```python
from build123d import *

# Parameters (mm, degrees)
PAD_DEPTH            = 42.5
SKETCH001_R          = 3.1
POCKET_DEPTH         = 27.001
POCKET_DEPTH_BACK    = -5.001
SKETCH002_R          = 2.6
SKETCH002_R_2        = 3.1
POCKET001_DEPTH      = 7.001
FILLET_R             = 2
SKETCH005_R          = 0.5
POCKET002_DEPTH      = 7.001
POCKET002_DEPTH_BACK = -27.001
SKETCH006_R          = 6
POCKET003_DEPTH      = 2


with BuildPart() as part:
    # Sketch → Pad (new body, symmetric)
    with BuildSketch(Plane.XZ):
        Polygon((-7, 5), (27, 5), (27, 0), (0, 0), (0, -27), (-7, -27), align=None)
    extrude(amount=PAD_DEPTH, both=True)

    # Sketch001 → Pocket (cut, two sides)
    with BuildSketch(Plane.XY) as pocket_sk:
        with Locations((15, -21)):
            Circle(SKETCH001_R)
        with Locations((15, 21)):
            Circle(SKETCH001_R)
    extrude(amount=-POCKET_DEPTH, mode=Mode.SUBTRACT)
    extrude(pocket_sk.sketch, amount=-POCKET_DEPTH_BACK, mode=Mode.SUBTRACT)

    # Sketch002 → Pocket001 (cut, through all)
    with BuildSketch(Plane.YZ):
        with Locations((-21, -15)):
            Circle(SKETCH002_R)
        with Locations((21, -15)):
            Circle(SKETCH002_R)
        with Locations((-35, -15)):
            Circle(SKETCH002_R_2)
        with Locations((35, -15)):
            Circle(SKETCH002_R_2)
    extrude(amount=-POCKET001_DEPTH, mode=Mode.SUBTRACT)

    # Sketch003 (on DatumPlane) → Groove (revolve, cut)
    with BuildSketch(Plane.XY.offset(-15)):
        Polygon((0, 21), (-5, 21), (0, 16), align=None)
    revolve(axis=Axis((0, 21, -15), (1, 0, 0)), mode=Mode.SUBTRACT)

    # Sketch004 (on DatumPlane) → Groove001 (revolve, cut)
    with BuildSketch(Plane.XY.offset(-15)):
        Polygon((-5, -21), (0, -21), (0, -16), align=None)
    revolve(axis=Axis((0, -21, -15), (1, 0, 0)), mode=Mode.SUBTRACT)

    # Fillet
    fillet_edges = [part.edges().sort_by_distance(p)[0] for p in [
        (-3.5, -42.5, -27),
        (-3.5, 42.5, -27),
        (10, -42.5, 5),
        (10, 42.5, 5),
    ]]
    fillet(fillet_edges, radius=FILLET_R)

    # Sketch005 → Pocket002 (cut, two sides)
    with BuildSketch(Plane.YZ) as pocket002_sk:
        with Locations((0, -27)):
            Circle(SKETCH005_R)
    extrude(amount=-POCKET002_DEPTH, mode=Mode.SUBTRACT)
    extrude(pocket002_sk.sketch, amount=-POCKET002_DEPTH_BACK, mode=Mode.SUBTRACT)

    # Sketch006 (on Face2 of Pocket002) → Pocket003 (cut)
    with BuildSketch(Plane(origin=(-7, 0, 0), x_dir=(0, 0, -1), z_dir=(-1, 0, 0))):
        with Locations((15, 35)):
            Circle(SKETCH006_R)
        with Locations((15, -35)):
            Circle(SKETCH006_R)
    extrude(amount=-POCKET003_DEPTH, mode=Mode.SUBTRACT)


solid = part.part
```
Check sheet for the modelled part. Datum: model origin and axes. Units: mm. A direction names the side the tool comes from. Round coordinates to 2 decimals unless told otherwise and drop trailing zeros. Write each loop counter-clockwise with the first axis right and the second up, starting at its lowest first coordinate (ties: lowest second). Pieces come first, ordered by that corner, then holes. Notation, with made-up numbers: (80.25, -9) -> (104.25, -9) arc R15 cw to (104.25, 9) -> close; hole circle Ø6 at (41.25, 33.25). An arc over 180 degrees is marked (long way). Put each result on its own line as item: value.
(1) Sectioned sample at C-C (y = -35). Enter the section's corners in (x, z).
Values found:
outline: (-7, -27) -> (0, -27) -> (0, -18.1) -> (-5, -18.1) -> (-5, -21) -> (-7, -21) -> close; (-7, -9) -> (-5, -9) -> (-5, -11.9) -> (0, -11.9) -> (0, 0) -> (27, 0) -> (27, 5) -> (-7, 5) -> close
(2) Sectioned sample at A-A (z = -15). Count the separate pieces of the cut face and the enclosed holes in it, plus the area to 3 significant figures.
Values found:
separate pieces: 5
enclosed holes: 0
area: 401 mm^2
(3) Sectioned sample at B-B (y = 21). Enter the section's corners in (x, z).
Values found:
outline: (-7, -27) -> (0, -27) -> (0, -20) -> (-2.4, -17.6) -> (-7, -17.6) -> close; (-7, -12.4) -> (-2.4, -12.4) -> (0, -10) -> (0, 0) -> (11.9, 0) -> (11.9, 5) -> (-7, 5) -> close; (18.1, 0) -> (27, 0) -> (27, 5) -> (18.1, 5) -> close
(4) Material ranges on line 1 (Y direction, x = 15, z = 1.1); line 2 (Y direction, x = -1.5, z = -13); line 3 (X direction, y = 28.5, z = -13.5), recorded low to high.
Values found:
line 1: y = -42.5 to -24.1, -17.9 to 17.9, 24.1 to 42.5
line 2: y = -42.5 to -37.37, -32.63 to -23.87, -18.13 to 18.13, 23.87 to 32.63, 37.37 to 42.5
line 3: x = -7 to 0
(5) Mould release check, pull along X, two halves, no side actions. Record for faces 1 (the face through (10.24, 41.9, 4.43)), 2 (the face through (14.328, -24.026, 2.465)), 3 (the face through (-2.25, 18.46, -13.95)): released by +X, released by -X, zero draft, split by the parting line, or undercut.
Values found:
face 1: zero draft
face 2: undercut
face 3: released by +X
(6) Go/stop test with flat-tipped pins: pin 1 Ø5.5 at (x, y) = (15, -21) entering from +Z; pin 2 Ø1.5 at (y, z) = (28, -18.5) entering from +X. Record where each tip stops, or that it passes through.
Values found:
pin 1: passes through
pin 2: stops at x = 0
(7) Tool access check on faces 4 (the face through (-1, 42.5, -7)), 5 (the face through (14, -1, 0)), 6 (the face through (-6.01, 37.3, -20.54)). Record the directions out of +Z, -Z, +X, -X, +Y, -Y that give a thin tool (end or side, any length) a straight path to the whole face; none if there is none.
Values found:
face 4: +Z, -Z, +X, -X, +Y
face 5: -Z, +X, +Y, -Y
face 6: -X
(8) Sectioned sample at D-D (x = 15). Enter the section's corners in (y, z), plus the area to 3 significant figures.
Values found:
outline: (-42.5, 0) -> (-24.1, 0) -> (-24.1, 5) -> (-40.5, 5) arc R2 ccw to (-42.5, 3) -> close; (-17.9, 0) -> (17.9, 0) -> (17.9, 5) -> (-17.9, 5) -> close; (24.1, 0) -> (42.5, 0) -> (42.5, 3) arc R2 ccw to (40.5, 5) -> (24.1, 5) -> close
area: 361 mm^2
